from build123d import *

# Parameters (mm, degrees)
F1_DEPTH = 20
F3_DEPTH = 150
F5_DEPTH = 50
F7_DEPTH = 54.463615
F9_DEPTH = 54.463615


with BuildPart() as f1:
    # F0 (on Front) → F1 (new body)
    with BuildSketch(Plane.XZ):
        Polygon((-28.408879, 27.231308), (-28.408879, 0), (-28.408879, -27.231308), (26.05374, -27.231308), (26.05374, 0), (26.05374, 27.231308), align=None)
    extrude(amount=F1_DEPTH)

    # F2 (on face) → F3 (join)
    with BuildSketch(Plane(origin=(0, 0, 0), x_dir=(-1, 0, 0), z_dir=(0, 1, 0))):
        Polygon((28.408879, -27.231308), (28.408879, 27.231308), (-26.05374, 27.231308), (-26.05374, 19.577103), (19.871499, 19.577103), (19.871499, 0), (19.871499, -19.577103), (-26.05374, -19.577103), (-26.05374, -27.231308), align=None)
    extrude(amount=F3_DEPTH)

    # F4 (on face) → F5 (join)
    with BuildSketch(Plane(origin=(-28.408879, 0, 0), x_dir=(0, -1, 0), z_dir=(-1, 0, 0))):
        Polygon((-150, 27.231308), (-150, 0), (-150, -27.231308), (-104.768693, -27.231308), (-104.768693, -19.577103), (-143.039733, -19.577103), (-143.039733, 0), (-143.039733, 19.577103), (-104.768693, 19.577103), (-104.768693, 27.231308), align=None)
    extrude(amount=F5_DEPTH)

    # F6 (on face) → F7 (cut, through all)
    with BuildSketch(Plane.XY.offset(27.231308)):
        Polygon((-14.289723, 87.620333), (26.05374, -8.034108), (26.05374, 150), (-14.289723, 150), align=None)
    extrude(amount=-F7_DEPTH, mode=Mode.SUBTRACT)

    # F8 (on face) → F9 (cut, through all)
    with BuildSketch(Plane.XY.offset(27.231308)):
        Polygon((-78.408879, 104.768693), (-28.408879, 104.768693), (-46.349301, 142.396316), (-78.408879, 142.396316), align=None)
    extrude(amount=-F9_DEPTH, mode=Mode.SUBTRACT)


solid = f1.part
Geometry: final body of the model. Coordinates: model frame, mm. A direction names the side the tool comes from. Round coordinates to 2 decimals unless told otherwise and drop trailing zeros. Loops run counter-clockwise (first coordinate to the right, second up) from the corner with the lowest first, then second, coordinate; pieces in that order, holes last. Notation, with made-up numbers: M 86.5,-39.75 L 104.5,-39.75 A17 ccw 104.5,-12.75 Z; hole C -22.75,15 d10. An arc over 180 degrees is marked long. Put each result on its own line as item: value. Start each with the question number.
(1) Material intervals for line 1 along Z through (x, y) = (-18.5, 129); line 2 along X through (y, z) = (15.5, -5.5); line 3 along Y through (x, z) = (-49, -13), sorted ascending. Write a range as [from, to].
(2) Section query A-A (x = 7.5). Return loops of the section in (y, z).
(3) Section query B-B (z = 8). Return loops of the section in (x, y), then the cut area to 3 significant figures.
(4) Contact query for flat-ended pins moving along their axis: pin 1 Ø8.5 at (y, z) = (131, 24.5) entering from +X; pin 2 Ø2 at (x, z) = (-31.5, 7.5) entering from -Y; pin 3 Ø16.5 at (y, z) = (96.5, -3.5) entering from -X. Output: stop coordinate, or through.
(5) Section query C-C (y = 3). Return loops of the section in (x, z), then the cut area to 3 significant figures.
(6) Draft query along Z for faces 5 (the face through (-19.871, 74, 0)), 6 (the face through (26.054, -14, 0)), 7 (the face through (-14, 53, -27.231)). Return one class per face: +Z half, -Z half, draft (parallel to the pull), parting line (faces both ways), or undercut.
(7) Section query D-D (y = 123.5). Return loops of the section in (x, z).
(8) Set-up query: faces 1 (the face through (-38, 131, 19.577)), 2 (the face through (-8, 41, 19.577)), 3 (the face through (-62, 142.396, -23)), 4 (the face through (-14.29, 119, -23)). Return all of +Z, -Z, +X, -X, +Y, -Y with unobstructed straight access to the full face (end or side cutting, diameter ignored); none if empty.
Findings below:
1. line 1: z = [-27.23, -19.58], [19.58, 27.23]
1. line 2: x = [-28.41, -19.87]
1. line 3: y = [143.04, 150]
2. outline: M -20,-27.23 L 35.96,-27.23 L 35.96,-19.58 L 0,-19.58 L 0,19.58 L 35.96,19.58 L 35.96,27.23 L -20,27.23 Z
3. outline: M -78.41,143.04 L -28.41,143.04 L -28.41,-20 L 26.05,-20 L 26.05,-8.03 L 22.67,0 L -19.87,0 L -19.87,150 L -78.41,150 Z
3. area: 2,700 mm2
4. pin 1: stops at x = -14.29
4. pin 2: stops at y = 143.04
4. pin 3: stops at x = -28.41
5. outline: M -28.41,-27.23 L 21.4,-27.23 L 21.4,-19.58 L -19.87,-19.58 L -19.87,19.58 L 21.4,19.58 L 21.4,27.23 L -28.41,27.23 Z
5. area: 1,100 mm2
6. face 5: undercut
6. face 6: draft
6. face 7: -Z half
7. outline: M -37.34,-27.23 L -14.29,-27.23 L -14.29,-19.58 L -19.87,-19.58 L -19.87,19.58 L -14.29,19.58 L -14.29,27.23 L -37.34,27.23 L -37.34,19.58 L -28.41,19.58 L -28.41,-19.58 L -37.34,-19.58 Z
8. face 1: -X, -Y
8. face 2: +X, +Y
8. face 3: +Z, -Z, -X, -Y
8. face 4: +Z, -Z, +X, +Y
